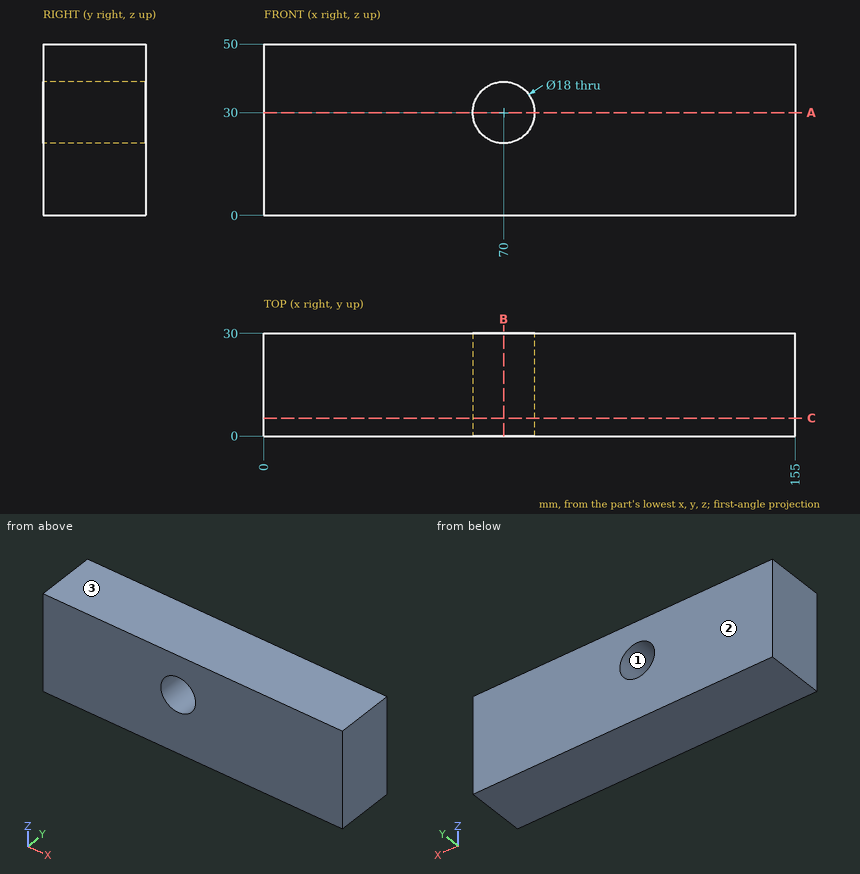
Could you check a few things on this drawing? It's one solid part, dimensions in mm from its lowest x, y, z. Round coordinates to 2 decimals unless told otherwise and drop trailing zeros. Write each loop counter-clockwise with the first axis right and the second up, starting at its lowest first coordinate (ties: lowest second). Pieces come first, ordered by that corner, then holes.
Q1. If we section it at B-B on x = 70: Write out the boundary of the cut face in (y, z), plus the area to 3 significant figures.
Q2. If we mould it in two halves opening along Z, with no side actions, what happens to the marked faces 1, 2 and 3? For each: +Z half, -Z half, draft (parallel to the pull), parting line (faces both ways), or undercut.
Q3. If we section it at A-A on z = 30: Write out the boundary of the cut face in (x, y).
Q4. Please list where these lines run through material, in increasing order: probe 1 along X at (y, z) = (6.5, 30); probe 2 along Z at (x, y) = (70, 10); probe 3 along X at (y, z) = (16, 24).
Q5. If we section it at C-C on y = 5.25: Write out the boundary of the cut face in (x, z).
Q6. Will this pin go through, and if not, where does the flat tip stop? P1, Ø4, axis at x = 24.5, z = 29.5, coming from the -Y side.
Answer below:
1. outline: (0, 0) - (30, 0) - (30, 21) - (0, 21) - close; (0, 39) - (30, 39) - (30, 50) - (0, 50) - close
1. area: 960 mm2
2. face 1: undercut
2. face 2: draft
2. face 3: +Z half
3. outline: (0, 0) - (61, 0) - (61, 30) - (0, 30) - close; (79, 0) - (155, 0) - (155, 30) - (79, 30) - close
4. probe 1: x = 0 to 61, 79 to 155
4. probe 2: z = 0 to 21, 39 to 50
4. probe 3: x = 0 to 63.29, 76.71 to 155
5. outline: (0, 0) - (155, 0) - (155, 50) - (0, 50) - close; hole circle Ø18 at (70, 30)
6. P1: stops at y = 0
